The drawing under review shows one solid part. Ordinate dimensions are in mm from its lowest x, y, z. Round coordinates to 2 decimals unless told otherwise and drop trailing zeros. Order: outer loops, then holes, each group sorted by start corner. A loop starts at its lowest first (then second) coordinate and runs counter-clockwise, first axis right, second up.
1) Clearance check with flat-ended pins moving along their axes: P1, Ø3, axis at x = 47, y = 6.5, coming from the -Z side; P2, Ø3, axis at x = 47.5, z = 23, coming from the +Y side; P3, Ø10, axis at y = 13.5, z = 9.5, coming from the -X side; P4, Ø10, axis at x = 17.5, y = 21.5, coming from the +Z side. State where each tip first meets the part, or that it passes through.
2) To check wall thickness, follow L1, parallel to Z at x = 13.5, y = 12; L2, parallel to X at y = 15.5, z = 34; L3, parallel to Z at x = 54, y = 7.5. State the ranges of each line that lie inside material, in increasing order.
3) Consider section C-C (y = 5.5). Give the boundary of the cut face in (x, z).
4) Consider section B-B (z = 33). Give the boundary of the cut face in (x, y).
5) Consider section A-A (x = 21.5). Give the boundary of the cut face in (y, z), then the cut area to 3 significant figures.
6) Consider section D-D (x = 46). Give the boundary of the cut face in (y, z), then the cut area to 3 significant figures.
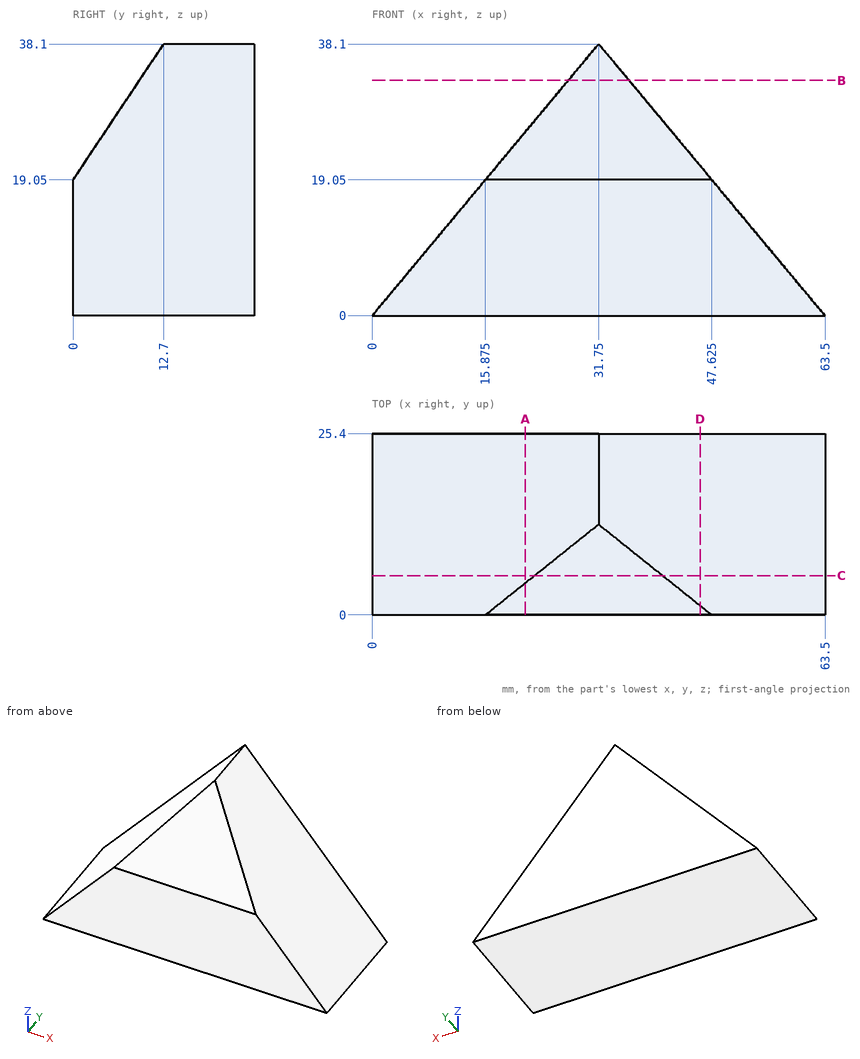
Answer below:
1. P1: stops at z = 0
1. P2: passes through
1. P3: stops at x = 3.75
1. P4: stops at z = 27
2. L1: z = 0 to 16.2
2. L2: x = 28.33 to 35.17
2. L3: z = 0 to 11.4
3. outline: (0, 0) - (63.5, 0) - (40.75, 27.3) - (22.75, 27.3) - close
4. outline: (27.5, 9.3) - (36, 9.3) - (36, 25.4) - (27.5, 25.4) - close
5. outline: (0, 0) - (25.4, 0) - (25.4, 25.8) - (4.5, 25.8) - (0, 19.05) - close
5. area: 640 mm2
6. outline: (0, 0) - (25.4, 0) - (25.4, 21) - (1.3, 21) - (0, 19.05) - close
6. area: 532 mm2
